Here's how the part is built. I have some questions about the finished solid (model axes, mm). Face numbers are marked on the shaded views. A direction names the side the tool comes from. Give positions to 0.01 mm unless a question says otherwise; leave off trailing zeros. Order: outer loops, then holes, each group sorted by start corner. A loop starts at its lowest first (then second) coordinate and runs counter-clockwise, first axis right, second up. Notation, with made-up numbers: M 20,31.5 L 70,31.5 A7 cw 70,36.5 Z; hole C -15,58.5 d6. An arc over 180 degrees is marked long. One line per item, written item: value. Start each with the question number.
from build123d import *

# Parameters (mm, degrees)
CUT_EXTRUDE1_START  = -8
CUT_EXTRUDE1_DEPTH  = 8
SKETCH4_W           = 8.5
SKETCH4_H           = 14
BOSS_EXTRUDE1_DEPTH = 4.9


with BuildPart() as part:
    # Sketch1 → Revolve5 (revolve)
    with BuildSketch(Plane(origin=(0, 0, 0), x_dir=(1, 0, 0), z_dir=(0, 1, 0))):
        Polygon((4.75, 4.5), (4.75, 12.1), (-65, 12.1), (-65, 10.1), (-55.5, 10.1), (-55.5, 8.6), (-53, 8.6), (-53, -0.35), (-31.9, -0.35), (-31.9, 0), (0, 0), (0, 4.5), align=None)
    revolve(axis=Axis((-65, 0, -12.1), (1, 0, 0)))

    # Sketch2 → Cut-Extrude1 (cut)
    with BuildSketch(Plane.ZY.offset(65).offset(CUT_EXTRUDE1_START)):
        with BuildLine():
            ThreePointArc((-10.6, -1.322875656), (-10.1, 0), (-10.6, 1.322875656))
            Line((-10.6, 1.322875656), (-10.6, -1.322875656))
        make_face()
    extrude(amount=CUT_EXTRUDE1_DEPTH, mode=Mode.SUBTRACT)

    # Sketch4 → Boss-Extrude1 (add)
    with BuildSketch(Plane(origin=(0, 0, 0), x_dir=(0, 0, -1), z_dir=(1, 0, 0))):
        with Locations((-0.75, 0)):
            Rectangle(SKETCH4_W, SKETCH4_H)
    extrude(amount=BOSS_EXTRUDE1_DEPTH)


solid = part.part
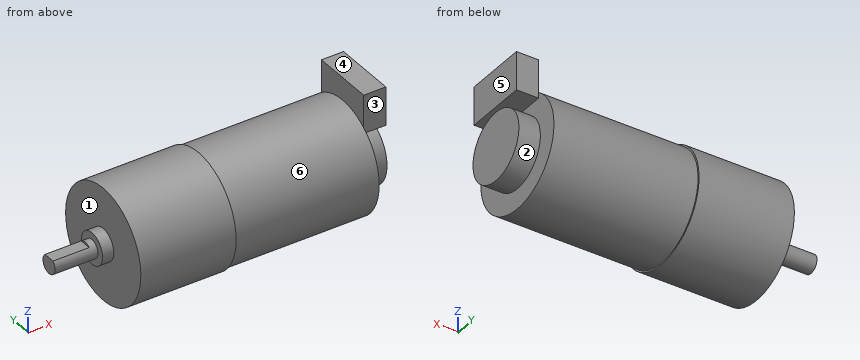
Item 1: I want a section at B-B on z = -12.1. Write out the boundary of the cut face in (x, y).
Item 2: I want a section at A-A on y = 0. Write out the boundary of the cut face in (x, z), plus the area to 3 significant figures.
Item 3: Please list where these lines run through material, in increasing order: probe 1 along X at (y, z) = (3.75, -0.5); probe 2 along X at (y, z) = (4, -18.25); probe 3 along X at (y, z) = (4, -18.75). Write a range as [from, to].
Item 4: I want a section at D-D on x = -8. Write out the boundary of the cut face in (y, z).
Item 5: I want a section at C-C on x = -43. Write out the boundary of the cut face in (y, z).
Item 6: We'd pull the mould along X, two halves only. Please class the marked faces 4, 5 and 6: +X half, -X half, draft (parallel to the pull), parting line (faces both ways), or undercut.
Item 7: For the marked faces 1, 2 and 3, which set-ups out of +Z, -Z, +X, -X, +Y, -Y let a thin tool reach every point of the face, with its end or its side?
Item 8: Will these pins go through, and if not, where does the flat tip stop? P1, Ø3, axis at y = -8.5, z = -17, coming from the +X side; P2, Ø4, axis at x = 2.5, z = -1, coming from the +Y side; P3, Ø3, axis at y = -6, z = -17, coming from the -X side; P4, Ø3, axis at y = -3, z = -11, coming from the -X side.
Answer below:
1. outline: M -65,-2 L -55.5,-2 L -55.5,-3.5 L -53,-3.5 L -53,-12.45 L -31.9,-12.45 L -31.9,-12.1 L 0,-12.1 L 0,-7.6 L 4.75,-7.6 L 4.75,7.6 L 0,7.6 L 0,12.1 L -31.9,12.1 L -31.9,12.45 L -53,12.45 L -53,3.5 L -55.5,3.5 L -55.5,2 L -65,2 Z
2. outline: M -65,-14.1 L -55.5,-14.1 L -55.5,-15.6 L -53,-15.6 L -53,-24.55 L -31.9,-24.55 L -31.9,-24.2 L 0,-24.2 L 0,-19.7 L 4.75,-19.7 L 4.75,-4.5 L 0,-4.5 L 0,-3.5 L 4.9,-3.5 L 4.9,5 L 0,5 L 0,0 L -31.9,0 L -31.9,0.35 L -53,0.35 L -53,-8.6 L -55.5,-8.6 L -55.5,-10.1 L -57,-10.1 L -57,-10.6 L -65,-10.6 Z
2. area: 1,460 mm²
3. probe 1: x = [-53, -31.9], [0, 4.9]
3. probe 2: x = [-53, 4.75]
3. probe 3: x = [-53, 0]
4. outline: C 0,-12.1 d24.2
5. outline: C 0,-12.1 d24.9
6. face 4: draft
6. face 5: +X half
6. face 6: undercut
7. face 1: -X
7. face 2: +X
7. face 3: +Z, +X, -Y
8. P1: stops at x = 0
8. P2: stops at y = 7
8. P3: stops at x = -53
8. P4: stops at x = -65
